Part model, mm, in its own coordinate system. Coordinates: 2 decimals unless noted, no trailing zeros. Loops run counter-clockwise (first coordinate to the right, second up) from the corner with the lowest first, then second, coordinate; pieces in that order, holes last. Notation, with made-up numbers: M 62,-19 L 92,-19 A16 cw 92,-8 Z; hole C 67.25,86.25 d3. An arc over 180 degrees is marked long. Answer as a JSON object with one key per item and string values. Group by question number.
1. Drop flat-ended pins along their axis: pin 1 Ø2.5 at (x, z) = (10.41, 47.56) entering from +Y; pin 2 Ø4 at (x, z) = (10.41, -30.15) entering from +Y (3 decimals); pin 3 Ø1.6 at (x, y) = (-14.5, 1.5) entering from -Z; pin 4 Ø1 at (x, y) = (-19.5, 1.5) entering from +Z. Give the stop position or say it passes through.
2. Saw through at C-C on y = 1.8. Count the separate pieces of the cut face and the enclosed holes in it, then the cut area to 3 significant figures.
3. Saw through at B-B on x = 15.5. Write the cut outline in (y, z) (3 decimals).
4. Saw through at A-A on x = 0. Write the cut outline in (y, z) (3 decimals).
5. Drill centre lines: L1, parallel to Z at x = -26, y = 1.85; L2, parallel to X at y = 1.9, z = 31; L3, parallel to X at y = 2.4, z = -18. Where is each one in solid material? Low to high.
6. Saw through at D-D on z = 43.5. Write the cut outline in (x, y) (3 decimals), then the cut area to 3 significant figures.
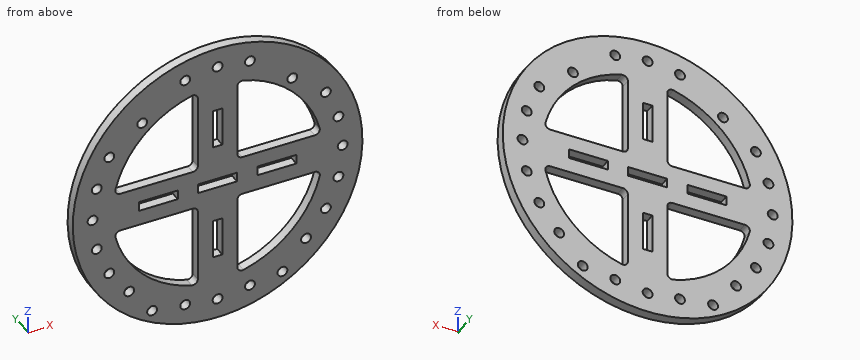
from build123d import *

# Parameters (mm, degrees)
SKETCH1_R           = 46.575911091
SKETCH1_R_2         = 1.587499996
SKETCH1_R_3         = 1.5875
SKETCH1_W           = 3.0226
SKETCH1_H           = 12.5476
SKETCH1_W_2         = 12.5476
SKETCH1_H_2         = 3.0226
SKETCH1_W_3         = 12.547600011
BOSS_EXTRUDE1_DEPTH = 3.175


with BuildPart() as part:
    # Sketch1 → Boss-Extrude1 (new body)
    with BuildSketch(Plane(origin=(0, 0, 0), x_dir=(1, 0, 0), z_dir=(0, 1, 0))):
        with Locations(Location((2.7e-08, -8.701819877, 0), (0, 0, 270))):
            Circle(SKETCH1_R)
        with Locations(Location((3e-08, 31.524091213, 0), (0, 0, 270))):
            Circle(SKETCH1_R_2, mode=Mode.SUBTRACT)
        with Locations(Location((-21.062340002, 28.785905516, 0), (0, 0, 270))):
            Circle(SKETCH1_R_3, mode=Mode.SUBTRACT)
        with Locations(Location((20.847659998, 28.785905516, 0), (0, 0, 270))):
            Circle(SKETCH1_R_3, mode=Mode.SUBTRACT)
        with Locations(Location((24.022659998, -37.254094484, 0), (0, 0, 270))):
            Circle(SKETCH1_R_3, mode=Mode.SUBTRACT)
        with Locations(Location((-24.237340002, -37.254094484, 0), (0, 0, 270))):
            Circle(SKETCH1_R_3, mode=Mode.SUBTRACT)
        with Locations(Location((10.411231927, 30.15342653, 0), (0, 0, 270))):
            Circle(SKETCH1_R_2, mode=Mode.SUBTRACT)
        with Locations(Location((28.444014541, 19.742194633, 0), (0, 0, 270))):
            Circle(SKETCH1_R_2, mode=Mode.SUBTRACT)
        with Locations(Location((34.836660923, 11.411135666, 0), (0, 0, 270))):
            Circle(SKETCH1_R_2, mode=Mode.SUBTRACT)
        with Locations(Location((38.855246436, 1.709412017, 0), (0, 0, 270))):
            Circle(SKETCH1_R_2, mode=Mode.SUBTRACT)
        with Locations(Location((40.225911118, -8.70181988, 0), (0, 0, 270))):
            Circle(SKETCH1_R_2, mode=Mode.SUBTRACT)
        with Locations(Location((38.855246435, -19.113051776, 0), (0, 0, 270))):
            Circle(SKETCH1_R_2, mode=Mode.SUBTRACT)
        with Locations(Location((34.836660921, -28.814775424, 0), (0, 0, 270))):
            Circle(SKETCH1_R_2, mode=Mode.SUBTRACT)
        with Locations(Location((10.411231922, -47.557066286, 0), (0, 0, 270))):
            Circle(SKETCH1_R_2, mode=Mode.SUBTRACT)
        with Locations(Location((2.5e-08, -48.927730968, 0), (0, 0, 270))):
            Circle(SKETCH1_R_2, mode=Mode.SUBTRACT)
        with Locations(Location((-10.411231872, -47.557066285, 0), (0, 0, 270))):
            Circle(SKETCH1_R_2, mode=Mode.SUBTRACT)
        with Locations(Location((-34.836660868, -28.81477542, 0), (0, 0, 270))):
            Circle(SKETCH1_R_2, mode=Mode.SUBTRACT)
        with Locations(Location((-38.855246381, -19.113051772, 0), (0, 0, 270))):
            Circle(SKETCH1_R_2, mode=Mode.SUBTRACT)
        with Locations(Location((-40.225911063, -8.701819875, 0), (0, 0, 270))):
            Circle(SKETCH1_R_2, mode=Mode.SUBTRACT)
        with Locations(Location((-38.85524638, 1.709412022, 0), (0, 0, 270))):
            Circle(SKETCH1_R_2, mode=Mode.SUBTRACT)
        with Locations(Location((-34.836660866, 11.41113567, 0), (0, 0, 270))):
            Circle(SKETCH1_R_2, mode=Mode.SUBTRACT)
        with Locations(Location((-28.444014482, 19.742194636, 0), (0, 0, 270))):
            Circle(SKETCH1_R_2, mode=Mode.SUBTRACT)
        with Locations(Location((-10.411231867, 30.153426532, 0), (0, 0, 270))):
            Circle(SKETCH1_R_2, mode=Mode.SUBTRACT)
        with BuildLine():
            Line((-6.349999989, -39.99938507), (-6.349999989, -16.639319886))
            ThreePointArc((-6.349999989, -16.639319886), (-6.814967973, -15.516787871), (-7.937499989, -15.051819886))
            Line((-7.937499989, -15.051819886), (-31.2975652, -15.051819886))
            ThreePointArc((-31.2975652, -15.051819886), (-32.55049963, -15.664480636), (-32.836349023, -17.029576972))
            ThreePointArc((-32.836349023, -17.029576972), (-23.953886478, -32.655706367), (-8.327757073, -41.538168895))
            ThreePointArc((-8.327757073, -41.538168895), (-6.962660738, -41.2523195), (-6.349999989, -39.99938507))
        make_face(mode=Mode.SUBTRACT)
        with Locations((1e-09, 10.348180116)):
            Rectangle(SKETCH1_W, SKETCH1_H, mode=Mode.SUBTRACT)
        with BuildLine():
            Line((6.350000022, -39.999385045), (6.350000022, -16.639319886))
            ThreePointArc((6.350000022, -16.639319886), (6.814968007, -15.516787871), (7.937500022, -15.051819886))
            Line((7.937500022, -15.051819886), (31.297565134, -15.051819886))
            ThreePointArc((31.297565134, -15.051819886), (32.550499564, -15.664480636), (32.836348958, -17.029576972))
            ThreePointArc((32.836348958, -17.029576972), (23.95388645, -32.655706329), (8.327757111, -41.538168868))
            ThreePointArc((8.327757111, -41.538168868), (6.962660773, -41.252319477), (6.350000022, -39.999385045))
        make_face(mode=Mode.SUBTRACT)
        with BuildLine():
            Line((-31.297565195, -2.351819884), (-7.937499989, -2.351819884))
            ThreePointArc((-7.937499989, -2.351819884), (-6.814967973, -1.886851899), (-6.349999989, -0.764319884))
            Line((-6.349999989, -0.764319884), (-6.349999989, 22.595745281))
            ThreePointArc((-6.349999989, 22.595745281), (-6.962660738, 23.848679711), (-8.327757073, 24.134529106))
            ThreePointArc((-8.327757073, 24.134529106), (-23.953886471, 15.252066585), (-32.836349018, -0.374062797))
            ThreePointArc((-32.836349018, -0.374062797), (-32.550499626, -1.739159134), (-31.297565195, -2.351819884))
        make_face(mode=Mode.SUBTRACT)
        with Locations((-19.049999999, -8.701819874)):
            Rectangle(SKETCH1_W_2, SKETCH1_H_2, mode=Mode.SUBTRACT)
        with Locations((1.7e-08, -8.701819874)):
            Rectangle(SKETCH1_W_3, SKETCH1_H_2, mode=Mode.SUBTRACT)
        with Locations((19.050000001, -8.701819874)):
            Rectangle(SKETCH1_W_2, SKETCH1_H_2, mode=Mode.SUBTRACT)
        with Locations((1e-09, -27.751819886)):
            Rectangle(SKETCH1_W, SKETCH1_H, mode=Mode.SUBTRACT)
        with BuildLine():
            Line((6.350000022, -0.764319884), (6.350000022, 22.595745256))
            ThreePointArc((6.350000022, 22.595745256), (6.962660773, 23.848679688), (8.327757111, 24.134529079))
            ThreePointArc((8.327757111, 24.134529079), (23.953886443, 15.252066547), (32.836348953, -0.374062797))
            ThreePointArc((32.836348953, -0.374062797), (32.55049956, -1.739159134), (31.297565129, -2.351819884))
            Line((31.297565129, -2.351819884), (7.937500022, -2.351819884))
            ThreePointArc((7.937500022, -2.351819884), (6.814968007, -1.886851899), (6.350000022, -0.764319884))
        make_face(mode=Mode.SUBTRACT)
    extrude(amount=BOSS_EXTRUDE1_DEPTH)


solid = part.part
Outcome:
{
 "1": {"pin 1": "passes through", "pin 2": "stops at y = 3.175", "pin 3": "stops at z = -35.81", "pin 4": "stops at z = 51.23"},
 "2": {"separate pieces": "1", "enclosed holes": "31", "area": "4,400 mm²"},
 "3": {"outline": "M 0,-35.219 L 3.175,-35.219 L 3.175,-21.42 L 0,-21.42 Z; M 0,2.352 L 3.175,2.352 L 3.175,7.191 L 0,7.191 Z; M 0,10.213 L 3.175,10.213 L 3.175,15.052 L 0,15.052 Z; M 0,38.824 L 3.175,38.824 L 3.175,52.623 L 0,52.623 Z"},
 "4": {"outline": "M 0,-37.874 L 3.175,-37.874 L 3.175,-33.112 L 0,-33.112 Z; M 0,-29.937 L 3.175,-29.937 L 3.175,-16.622 L 0,-16.622 Z; M 0,-4.074 L 3.175,-4.074 L 3.175,7.191 L 0,7.191 Z; M 0,10.213 L 3.175,10.213 L 3.175,21.478 L 0,21.478 Z; M 0,34.026 L 3.175,34.026 L 3.175,47.34 L 0,47.34 Z; M 0,50.515 L 3.175,50.515 L 3.175,55.278 L 0,55.278 Z"},
 "5": {"L1": "z = -29.94 to -13.01, 2.35 to 15.05, 30.42 to 47.35", "L2": "x = -40.89 to -25.5, -6.35 to -1.51, 1.51 to 6.35, 25.5 to 40.89", "L3": "x = -38.16 to -20.85, -6.35 to 6.35, 20.85 to 38.16"},
 "6": {"outline": "M -30.958,0 L 30.958,0 L 30.958,3.175 L -30.958,3.175 Z", "area": "197 mm²"}
}
